Design review of the part built by this model. Coordinates are the model's own, in mm. A direction names the side the tool comes from. Coordinates: 2 decimals unless noted, no trailing zeros. Write each loop counter-clockwise with the first axis right and the second up, starting at its lowest first coordinate (ties: lowest second). Pieces come first, ordered by that corner, then holes.
Q1. For faces 4 (the cylindrical face through (24.976, 149.413, -1.099)), 5 (the flat face through (-85, 79, 36)), 6 (the cylindrical face through (-69, 10, 0)), 7 (the flat face through (0, 185, 11)), list the 3-axis set-ups (+Z, -Z, +X, -X, +Y, -Y) from which the entire face can be reached by the end or side of a thin tool; tool diameter is ignored.
Q2. For pin 1 Ø11 at (x, z) = (-63, 0) entering from +Y; pin 2 Ø6 at (x, y) = (-64.5, 108.5) entering from +Z; pin 3 Ø8 at (y, z) = (96.5, 3) entering from +X; pin 4 Ø9.5 at (y, z) = (159.55, -44.55) entering from -X, all flat-tipped, find the tip position at first contact; note any pin that passes through.
Q3. The part is to be moulded in two halves that separate along Y. For faces 1 (the cylindrical face through (-50.54, 9.86, -44.28)), 2 (the cylindrical face through (-97.68, 119.06, 58.58)), 3 (the cylindrical face through (-97.675, 196.798, -10.74)), say which applies: released by +Y, released by -Y, zero draft, split by the parting line, or undercut.
Q4. For L1, parallel to Z at x = 0, y = 6; L2, parallel to Z at x = 0, y = 129.5; L3, parallel to Y at x = -73, z = -21, list the stretches that pass through material, from the lowest coordinate up.
Q5. Take a section at B-B, the plane x = 63. Write out the cut boundary in (y, z).
Q6. Take a section at C-C, the plane x = -46. State how many separate pieces and enclosed holes the cut face has, plus the area to 3 significant figures.
Q7. Take a section at A-A, the plane z = 72.5. Write out the cut boundary in (x, y), plus the area to 3 significant figures.
from build123d import *

# Parameters (mm, degrees)
SKETCH6_R           = 43
SKETCH6_R_2         = 27
BOSS_EXTRUDE1_REACH = 187
SKETCH7_R           = 25
CUT_EXTRUDE1_REACH  = 187
SKETCH8_R           = 10
SKETCH9_R           = 82.5
BOSS_EXTRUDE2_DEPTH = 20
SKETCH10_R          = 27
CUT_EXTRUDE2_DEPTH  = 20
SKETCH11_R          = 6
CUT_EXTRUDE3_DEPTH  = 20
SKETCH12_R          = 82.5
BOSS_EXTRUDE3_DEPTH = 25
SKETCH13_R          = 6
CUT_EXTRUDE4_DEPTH  = 25
SKETCH14_R          = 27
CUT_EXTRUDE5_DEPTH  = 25


with BuildPart() as part:
    # Sweep-Thin1: sweep along a path in Sketch5
    with BuildLine(Plane.XY) as sweep_thin1_path:
        Line((0, 0), (0, 25))
        ThreePointArc((0, 25), (-26.360389693, 88.639610307), (-90, 115))
        Line((-90, 115), (-110, 115))
    # Sketch6 → Sweep-Thin1 (sweep)
    with BuildSketch(Plane(origin=(0, 0, 0), x_dir=(1, 0, 0), z_dir=(0, 1, 0))):
        Circle(SKETCH6_R)
        Circle(SKETCH6_R_2, mode=Mode.SUBTRACT)
    sweep(path=sweep_thin1_path.line)

    # Sketch7 → Boss-Extrude1 (add, up to next)
    with BuildSketch(Plane(origin=(0, 185, 0), x_dir=(-1, 0, 0), z_dir=(0, -1, 0)), mode=Mode.PRIVATE) as boss_extrude1_sk1:
        Circle(SKETCH7_R)
    boss_extrude1_tool1 = extrude(boss_extrude1_sk1.sketch, amount=BOSS_EXTRUDE1_REACH, mode=Mode.PRIVATE) - part.part
    add(boss_extrude1_tool1.solids().sort_by_distance((0, 185, 0))[0])

    # Sketch8 → Cut-Extrude1 (cut, up to next)
    with BuildSketch(Plane(origin=(0, 185, 0), x_dir=(1, 0, 0), z_dir=(0, 1, 0)), mode=Mode.PRIVATE) as cut_extrude1_sk1:
        Circle(SKETCH8_R)
    cut_extrude1_tool1 = extrude(cut_extrude1_sk1.sketch, amount=-CUT_EXTRUDE1_REACH, mode=Mode.PRIVATE) & part.part
    add(cut_extrude1_tool1.solids().sort_by_distance((0, 185, 0))[0], mode=Mode.SUBTRACT)

    # Sketch9 → Boss-Extrude2 (add)
    with BuildSketch(Plane.XZ):
        Circle(SKETCH9_R)
    extrude(amount=-BOSS_EXTRUDE2_DEPTH)

    # Sketch10 → Cut-Extrude2 (cut)
    with BuildSketch(Plane.XZ):
        Circle(SKETCH10_R)
    extrude(amount=-CUT_EXTRUDE2_DEPTH, mode=Mode.SUBTRACT)

    # Sketch11 → Cut-Extrude3 (cut)
    with BuildSketch(Plane.XZ):
        with Locations((-63, 0)):
            Circle(SKETCH11_R)
        with Locations((-44.547727215, 44.547727215)):
            Circle(SKETCH11_R)
        with Locations((0, 63)):
            Circle(SKETCH11_R)
        with Locations((44.547727215, 44.547727215)):
            Circle(SKETCH11_R)
        with Locations((63, 0)):
            Circle(SKETCH11_R)
        with Locations((44.547727215, -44.547727215)):
            Circle(SKETCH11_R)
        with Locations((0, -63)):
            Circle(SKETCH11_R)
        with Locations((-44.547727215, -44.547727215)):
            Circle(SKETCH11_R)
    extrude(amount=-CUT_EXTRUDE3_DEPTH, mode=Mode.SUBTRACT)

    # Sketch12 → Boss-Extrude3 (add)
    with BuildSketch(Plane.ZY.offset(110)):
        with Locations((0, 115)):
            Circle(SKETCH12_R)
    extrude(amount=-BOSS_EXTRUDE3_DEPTH)

    # Sketch13 → Cut-Extrude4 (cut)
    with BuildSketch(Plane.ZY.offset(110)):
        with Locations((-63, 115)):
            Circle(SKETCH13_R)
        with Locations((-44.547727215, 159.547727215)):
            Circle(SKETCH13_R)
        with Locations((0, 178)):
            Circle(SKETCH13_R)
        with Locations((44.547727215, 159.547727215)):
            Circle(SKETCH13_R)
        with Locations((63, 115)):
            Circle(SKETCH13_R)
        with Locations((44.547727215, 70.452272785)):
            Circle(SKETCH13_R)
        with Locations((0, 52)):
            Circle(SKETCH13_R)
        with Locations((-44.547727215, 70.452272785)):
            Circle(SKETCH13_R)
    extrude(amount=-CUT_EXTRUDE4_DEPTH, mode=Mode.SUBTRACT)

    # Sketch14 → Cut-Extrude5 (cut)
    with BuildSketch(Plane.ZY.offset(110)):
        with Locations((0, 115)):
            Circle(SKETCH14_R)
    extrude(amount=-CUT_EXTRUDE5_DEPTH, mode=Mode.SUBTRACT)


solid = part.part
Responses:
1. face 4: +Y
1. face 5: none
1. face 6: -Y
1. face 7: +Z, -Z, +X, +Y
2. pin 1: stops at y = 156.25
2. pin 2: stops at z = 43
2. pin 3: stops at x = 25
2. pin 4: passes through
3. face 1: zero draft
3. face 2: undercut
3. face 3: split by the parting line
4. L1: z = -82.5 to -69, -57 to -27, 27 to 57, 69 to 82.5
4. L2: z = -25 to -10, 10 to 25
4. L3: y = 0 to 20, 74.65 to 96.02, 130.61 to 151.39
5. outline: (0, -53.27) - (20, -53.27) - (20, -6) - (0, -6) - close; (0, 6) - (20, 6) - (20, 53.27) - (0, 53.27) - close
6. separate pieces: 4
6. enclosed holes: 1
6. area: 6,700 mm2
7. outline: (-110, 75.63) - (-85, 75.63) - (-85, 154.37) - (-110, 154.37) - close; (-39.37, 0) - (39.37, 0) - (39.37, 20) - (-39.37, 20) - close
7. area: 3,540 mm2
